from build123d import *

# Parameters (mm, degrees)
ESQUISSE2_OUTSIDE_W     = 386.766
ESQUISSE2_OUTSIDE_H     = 238.266
ESQUISSE2_OUTSIDE_W_2   = 228
ESQUISSE2_OUTSIDE_H_2   = 155
ENL_V_MAT_EXTRU_1_DEPTH = 150
ENL_V_MAT_EXTRU_2_DEPTH = 239.646705404
BOSS_EXTRU_1_DEPTH      = 3
BOSS_EXTRU_2_START      = -3
BOSS_EXTRU_2_DEPTH      = 3
CONG_9_R                = 3


with BuildPart() as part:
    # Esquisse1 → Révolution4 (revolve)
    with BuildSketch(Plane.XY, mode=Mode.PRIVATE) as r_volution4_sk:
        with BuildLine():
            Line((148, 12.175795662), (148, 1))
            Line((148, 1), (145, 1))
            Line((145, 1), (145, 12.051970793))
            ThreePointArc((145, 12.051970793), (98.530929788, 107.060290842), (0, 145.5))
            Line((0, 145.5), (0, 148.5))
            ThreePointArc((0, 148.5), (100.608509442, 109.225353412), (148, 12.175795662))
        make_face()
    revolve(r_volution4_sk.sketch.rotate(Axis((0, 0, 0), (0, 1, 0)), 90), axis=Axis((0, 0, 0), (0, 1, 0)))

    # Esquisse2 outside → Enlèv. mat.-Extru.1 (cut, symmetric)
    with BuildSketch(Plane.XY):
        with Locations((0, 74.75)):
            Rectangle(ESQUISSE2_OUTSIDE_W, ESQUISSE2_OUTSIDE_H)
        with Locations((0, 72.5)):
            Rectangle(ESQUISSE2_OUTSIDE_W_2, ESQUISSE2_OUTSIDE_H_2, mode=Mode.SUBTRACT)
    extrude(amount=ENL_V_MAT_EXTRU_1_DEPTH, both=True, mode=Mode.SUBTRACT)

    # Esquisse3 → Enlèv. mat.-Extru.2 (cut, through all)
    with BuildSketch(Plane(origin=(0, 0, 0), x_dir=(1, 0, 0), z_dir=(0, 1, 0))):
        with BuildLine():
            Line((-25, -20), (-25, 20))
            ThreePointArc((-25, 20), (0, 45), (25, 20))
            Line((25, 20), (25, -20))
            ThreePointArc((25, -20), (0, -45), (-25, -20))
        make_face()
    extrude(amount=ENL_V_MAT_EXTRU_2_DEPTH, mode=Mode.SUBTRACT)

    # Esquisse4 → Boss.-Extru.1 (add)
    with BuildSketch(Plane(origin=(114, 0, 0), x_dir=(0, 0, -1), z_dir=(1, 0, 0))):
        with BuildLine():
            Line((-93.994680701, 1), (-74.993333037, 1))
            ThreePointArc((-74.993333037, 1), (0, 75), (74.993333037, 1))
            Line((74.993333037, 1), (93.994680701, 1))
            ThreePointArc((93.994680701, 1), (0, 94), (-93.994680701, 1))
        make_face()
    extrude(amount=-BOSS_EXTRU_1_DEPTH)

    # Esquisse5 → Boss.-Extru.2 (add)
    with BuildSketch(Plane.ZY.offset(114).offset(BOSS_EXTRU_2_START)):
        with BuildLine():
            Line((-93.994680701, 1), (-74.993333037, 1))
            ThreePointArc((-74.993333037, 1), (0, 75), (74.993333037, 1))
            Line((74.993333037, 1), (93.994680701, 1))
            ThreePointArc((93.994680701, 1), (0, 94), (-93.994680701, 1))
        make_face()
    extrude(amount=BOSS_EXTRU_2_DEPTH)

    # Congé9
    # the kernel refuses this fillet: 3 mm, written as the material it takes off along each edge
    with BuildSketch(Plane(origin=(-114, 20.411983352, -94.382201712), x_dir=(0.6405708887604551, 0, -0.767899040546764), z_dir=(0, -1, 0)), Plane(origin=(114, 20.411983352, 94.382201712), x_dir=(-0.6405708887604538, 0, 0.7678990405467649), z_dir=(0, -1, 0))) as cong_9_piece_1:
        with BuildLine():
            CenterArc((1.087028375, 2.999979354), CONG_9_R, 230.165597581, 40.046969931)
            Line((-0.834684291, 0.696282232), (0, 0))
            ThreePointArc((0, 0), (0.549079179, -0.001018544), (1.098158359, 0))
        make_face()
    extrude(amount=22.157379249, mode=Mode.SUBTRACT)
    with BuildSketch(Plane(origin=(-114, 0, 0), x_dir=(0, 0.09906318090270165, -0.9950811455300712), z_dir=(0, -0.9950811455300712, -0.09906318090270165))) as cong_9_piece_2:
        with BuildLine():
            CenterArc((94.070452322, 3), CONG_9_R, 270, 40.28066089)
            ThreePointArc((96.010049277, 0.711340206), (95.587852119, 0.354883399), (95.164331553, 0))
            Line((95.164331553, 0), (94.070452322, 0))
        make_face()
    revolve(axis=Axis((-114, 0, 0), (1, 0, 0)), revolution_arc=168.629546335, mode=Mode.SUBTRACT)
    with BuildSketch(Plane(origin=(-114, 20.411983352, 94.382201712), x_dir=(0, 0, -1), z_dir=(0, -1, 0))) as cong_9_piece_3:
        with BuildLine():
            CenterArc((1.086971394, 3), CONG_9_R, 229.953030069, 40.046969931)
            ThreePointArc((-0.84327475, 0.703448276), (-0.422289825, 0.350941999), (0, 0))
            Line((0, 0), (1.086971394, 0))
        make_face()
    extrude(amount=22.157379249, mode=Mode.SUBTRACT)
    with BuildSketch(Plane(origin=(114, 0, 0), x_dir=(0, 0.09906318090270108, 0.9950811455300712), z_dir=(0, -0.9950811455300712, 0.09906318090270108))) as cong_9_piece_4:
        with BuildLine():
            CenterArc((94.070452322, 3), CONG_9_R, 270, 40.28066089)
            Line((94.070452322, 0), (95.164331553, 0))
            ThreePointArc((95.164331553, 0), (95.587852119, 0.354883399), (96.010049277, 0.711340206))
        make_face()
    revolve(axis=Axis((114, 0, 0), (-1, 0, 0)), revolution_arc=168.629546335, mode=Mode.SUBTRACT)
    with BuildSketch(Plane(origin=(114, 20.411983352, -94.382201712), x_dir=(-0.6405708887604424, 0, -0.7678990405467746), z_dir=(0, -1, 0))) as cong_9_piece_5:
        with BuildLine():
            CenterArc((1.087028375, -2.999979354), CONG_9_R, 89.787432488, 40.046969931)
            Line((-0.834684291, -0.696282232), (0, 0))
            ThreePointArc((0, 0), (0.549079179, 0.001018544), (1.098158359, 0))
        make_face()
    extrude(amount=22.157379249, mode=Mode.SUBTRACT)


solid = part.part
Here's how the part is built. I have some questions about the finished solid (model axes, mm). A direction names the side the tool comes from. Coordinates: 2 decimals unless noted, no trailing zeros. Loops run counter-clockwise (first coordinate to the right, second up) from the corner with the lowest first, then second, coordinate; pieces in that order, holes last. Notation, with made-up numbers: (-28.75, 25) -> (-17.75, 25) arc R24 cw to (-17.75, 46) -> close; hole circle Ø4 at (45.25, 67.25). An arc over 180 degrees is marked (long way). Use one line per item in the form item = value. Start each with the question number.
(1) If we section it at A-A (x = 15): Please give me the cut outline in (y, z), then the cut area to 3 significant figures.
(2) On a 3-axis mill with a long thin cutter (end or side, diameter ignored), from which of +Z, -Z, +X, -X, +Y, -Y can I reach the whole of each face in a straight line? I mean faces 1 (the face through (111, 79, -6)), 2 (the face through (0.55, 140.902, 44.994)), 3 (the face through (114, 78, 0)). Say none if no direction works.
(3) If we section it at C-C (z = 101): Please give me the cut outline in (x, y).
(4) Will these pins go through, and if not, where does the flat tip stop? pin 1 (12 mm diameter, centred on x = 26, y = 21.5, fed in from +Z); pin 2 (1.5 mm diameter, centred on x = -71.5, z = -69.5, fed in from -Y); pin 3 (6 mm diameter, centred on x = -60.5, y = 97.5, fed in from +Z).
(5) Please list where these lines run through material, in increasing order: line 1 along X through (y, z) = (7, 83); line 2 along Z through (x, y) = (44, 41); line 3 along Z through (x, y) = (-1, 43.5).
(6) If we section it at B-B (x = 66): Please give me the cut outline in (y, z).
Verdict:
q1.outline = (1, -147.24) -> (12.18, -147.24) arc R147.74 ccw to (142.22, -40) -> (139.09, -40) arc R144.72 cw to (12.05, -144.22) -> (1, -144.22) -> close; (1, 144.22) -> (12.05, 144.22) arc R144.72 cw to (139.09, 40) -> (142.22, 40) arc R147.74 ccw to (12.18, 147.24) -> (1, 147.24) -> close
q1.area = 1,130 mm²
q2.face_1 = -Y
q2.face_2 = +Y, -Y
q2.face_3 = +Z, -Z, +X, +Y, -Y
q3.outline = (-108.18, 1) -> (-104.04, 1) -> (-104.04, 12.05) arc R104.73 cw to (104.04, 12.05) -> (104.04, 1) -> (108.18, 1) -> (108.18, 12.18) arc R108.86 ccw to (-108.18, 12.18) -> close
q4.pin_1 = 145.89
q4.pin_2 = 105.25
q4.pin_3 = 97.8
q5.line_1 = -114 to -111, 111 to 114
q5.line_2 = -135.78 to -132.49, 132.49 to 135.78
q5.line_3 = -141.98 to -138.84, 138.84 to 141.98
q6.outline = (1, -132.47) -> (12.18, -132.47) arc R133.03 ccw to (12.18, 132.47) -> (1, 132.47) -> (1, 129.11) -> (12.05, 129.11) arc R129.67 cw to (12.05, -129.11) -> (1, -129.11) -> close
